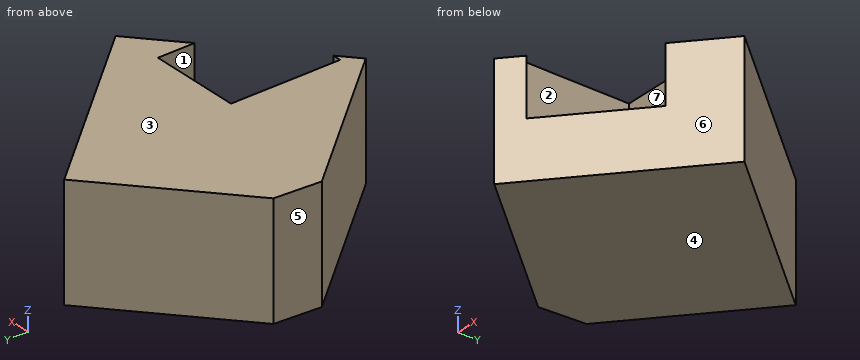
```python
from build123d import *

# Parameters (mm, degrees)
F1_DEPTH = 50.8
F2_W     = 40.923903
F2_H     = 48.857377
F3_DEPTH = 25.4


with BuildPart() as f1:
    # F0 (on Top) → F1 (new body)
    with BuildSketch(Plane.XY):
        Polygon((0, 67.501426), (-55.901939, 18.58723), (-57.277205, -2.041763), (0, -67.501426), (66.904068, -8.960366), align=None)
    extrude(amount=F1_DEPTH)

    # F2 (on face) → F3 (cut)
    with BuildSketch(Plane.XY.offset(50.8)):
        with Locations((25.341062, -35.488515)):
            Rectangle(F2_W, F2_H)
    extrude(amount=-F3_DEPTH, mode=Mode.SUBTRACT)


solid = f1.part
```
Build history of the part. All positions in model axes, mm. Face numbers are marked on the shaded views. A direction names the side the tool comes from. Give positions to 0.01 mm unless a question says otherwise; leave off trailing zeros. Loops run counter-clockwise (first coordinate to the right, second up) from the corner with the lowest first, then second, coordinate; pieces in that order, holes last.
1) Band-saw the part on A-A on z = 43. List the corners of the cut face in (x, y).
Values follow:
outline: (-57.28, -2.04) - (0, -67.5) - (8.67, -59.92) - (4.88, -59.92) - (4.88, -11.06) - (45.8, -11.06) - (45.8, -27.42) - (66.9, -8.96) - (0, 67.5) - (-55.9, 18.59) - close
2) Two-plate mould, pull along X, no slides. Class the marked faces 4, 5, 6 and 7: released by +X, released by -X, zero draft, split by the parting line, or undercut.
Values follow:
face 4: zero draft
face 5: released by -X
face 6: released by +X
face 7: undercut
3) Band-saw the part on C-C on y = -54. List the corners of the cut face in (x, z), then the cut area to 3 significant figures.
Values follow:
outline: (-11.81, 0) - (15.43, 0) - (15.43, 25.4) - (4.88, 25.4) - (4.88, 50.8) - (-11.81, 50.8) - close
area: 1,120 mm2
4) 3-axis set-ups, long thin cutter, end or side, ignore diameter. For the marked faces 1, 2 and 3: which of +Z, -Z, +X, -X, +Y, -Y reach the whole face in a straight line?
Values follow:
face 1: +Z, -Y
face 2: +Z
face 3: +Z, +X, -X, +Y, -Y
5) Drop flat-ended pins along their axis: P1, Ø7.5, axis at x = 30, z = 43, coming from the -Y side; P2, Ø1, axis at y = -28, z = 31.5, coming from the +X side; P3, Ø1.9, axis at x = 7, z = 44.5, coming from the +Y side. Give the stop position or say it passes through.
Values follow:
P1: stops at y = -11.06
P2: stops at x = 4.88
P3: stops at y = 60.59
6) Probe line 1 along X through (y, z) = (-22.5, 30.5); line 2 along Y through (x, z) = (-20, 17); line 3 along X through (y, z) = (-16, 32.5). List the from-to ranges inside material, lowest first.
Values follow:
line 1: x = -39.38 to 4.88, 45.8 to 51.43
line 2: y = -44.64 to 50
line 3: x = -45.06 to 4.88, 45.8 to 58.86
7) Band-saw the part on B-B on x = 20.5. List the corners of the cut face in (y, z), then the cut area to 3 significant figures.
Values follow:
outline: (-49.56, 0) - (44.07, 0) - (44.07, 50.8) - (-11.06, 50.8) - (-11.06, 25.4) - (-49.56, 25.4) - close
area: 3,780 mm2
8) Band-saw the part on D-D on z = 8. List the corners of the cut face in (x, y).
Values follow:
outline: (-57.28, -2.04) - (0, -67.5) - (66.9, -8.96) - (0, 67.5) - (-55.9, 18.59) - close
